Check sheet for the modelled part. Datum: model origin and axes. Units: mm. Face numbers are marked on the shaded views. A direction names the side the tool comes from. Round coordinates to 2 decimals unless told otherwise and drop trailing zeros. Write each loop counter-clockwise with the first axis right and the second up, starting at its lowest first coordinate (ties: lowest second). Pieces come first, ordered by that corner, then holes. Notation, with made-up numbers: M 66,24.25 L 88,24.25 A12 ccw 88,39.25 Z; hole C -10,39 d5. An arc over 180 degrees is marked long. Put each result on its own line as item: value.
```python
from build123d import *

# Parameters (mm, degrees)
F0_W     = 19
F0_H     = 19
F1_DEPTH = 2
F3_DEPTH = 8
F4_R     = 5
F5_R     = 1


with BuildPart() as f1:
    # F0 (on Top) → F1 (new body)
    with BuildSketch(Plane.XY):
        Rectangle(F0_W, F0_H)
    extrude(amount=F1_DEPTH)

    # F2 (on face) → F3 (join)
    with BuildSketch(Plane.XY.offset(2)):
        with BuildLine():
            Line((9.5, -4.25), (6.3307286311, -4.25))
            ThreePointArc((6.3307286311, -4.25), (0, -7.625), (-6.3307286311, -4.25))
            Line((-6.3307286311, -4.25), (-9.5, -4.25))
            Line((-9.5, -4.25), (-9.5, -9.5))
            Line((-9.5, -9.5), (9.5, -9.5))
            Line((9.5, -9.5), (9.5, -4.25))
        make_face()
        with BuildLine():
            ThreePointArc((-6.3307286311, 4.25), (0, 7.625), (6.3307286311, 4.25))
            Line((6.3307286311, 4.25), (9.5, 4.25))
            Line((9.5, 4.25), (9.5, 9.5))
            Line((9.5, 9.5), (-9.5, 9.5))
            Line((-9.5, 9.5), (-9.5, 4.25))
            Line((-9.5, 4.25), (-6.3307286311, 4.25))
        make_face()
    extrude(amount=F3_DEPTH)

    # F4
    f4_edges = [f1.edges().sort_by_distance(p)[0] for p in [
        (-9.5, -9.5, 5),
        (9.5, -9.5, 5),
        (9.5, 9.5, 5),
        (-9.5, 9.5, 5),
    ]]
    fillet(f4_edges, radius=F4_R)

    # F5
    f5_edges = [f1.edges().sort_by_distance(p)[0] for p in [
        (6.330729, 4.25, 6),
        (-6.330729, 4.25, 6),
        (-6.330729, -4.25, 6),
    ]]
    fillet(f5_edges, radius=F5_R)


solid = f1.part
```
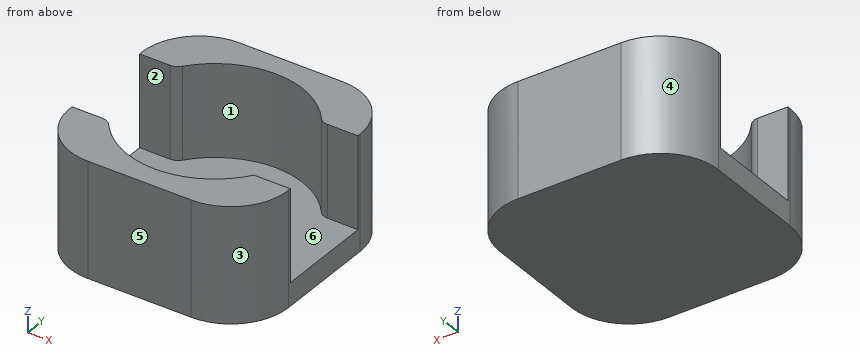
1. Release check for a two-part mould opening along Y. For the marked faces 4, 5 and 6 record: +Y half, -Y half, draft (parallel to the pull), parting line (faces both ways), or undercut.
Computed values:
face 4: +Y half
face 5: -Y half
face 6: undercut
2. Cross-section at A-A (z = 8). Enter the section's corners in (x, y) (3 decimals).
Computed values:
outline: M -9.5,-4.5 A5 ccw -4.5,-9.5 L 4.5,-9.5 A5 ccw 9.5,-4.5 L 9.5,-4.25 L 6.331,-4.25 A7.625 cw -6.05,-4.641 A1 ccw -6.843,-4.25 L -9.5,-4.25 Z; M -9.5,4.25 L -6.843,4.25 A1 ccw -6.05,4.641 A7.625 cw 6.05,4.641 A1 ccw 6.843,4.25 L 9.5,4.25 L 9.5,4.5 A5 ccw 4.5,9.5 L -4.5,9.5 A5 ccw -9.5,4.5 Z
3. Depth check by flat-ended pin: pin 1 Ø1.5 at (x, y) = (3, -0.5) entering from +Z; pin 2 Ø0.8 at (x, z) = (8, 7.5) entering from -Y; pin 3 Ø6 at (x, z) = (-7, 2) entering from -Y; pin 4 Ø0.8 at (x, z) = (-8, 8) entering from +Y. Enter the tip coordinate at first touch or a pass-through.
Computed values:
pin 1: stops at z = 2
pin 2: stops at y = -8.42
pin 3: stops at y = -9.5
pin 4: stops at y = 8.42
4. Cross-section at B-B (z = 1.75). Enter the section's corners in (x, y).
Computed values:
outline: M -9.5,-4.5 A5 ccw -4.5,-9.5 L 4.5,-9.5 A5 ccw 9.5,-4.5 L 9.5,4.5 A5 ccw 4.5,9.5 L -4.5,9.5 A5 ccw -9.5,4.5 Z
5. Cross-section at C-C (x = 8.5). Enter the section's corners in (y, z), then the cut area to 3 significant figures.
Computed values:
outline: M -7.5,0 L 7.5,0 L 7.5,10 L 4.25,10 L 4.25,2 L -4.25,2 L -4.25,10 L -7.5,10 Z
area: 82.0 mm2
6. Scan lines: probe 1 along Z at (x, y) = (2, -3); probe 2 along Y at (x, z) = (5.25, 3); probe 3 along Y at (x, z) = (6.75, 7.25). Record each from-to range of solid material in increasing order.
Computed values:
probe 1: z = 0 to 2
probe 2: y = -9.44 to -5.53, 5.53 to 9.44
probe 3: y = -8.97 to -4.25, 4.25 to 8.97
7. Cross-section at D-D (y = -0.5). Enter the section's corners in (x, z).
Computed values:
outline: M -9.5,0 L 9.5,0 L 9.5,2 L -9.5,2 Z
8. Access from +Z, -Z, +X, -X, +Y, -Y to the whole of each face (thin tool, end or side, straight path). Record for the marked faces 1, 2 and 3.
Computed values:
face 1: +Z
face 2: +Z, +X, -X
face 3: +Z, -Z, +X, -Y
